Design review of the part built by this model. Coordinates are the model's own, in mm. A direction names the side the tool comes from. Give positions to 0.01 mm unless a question says otherwise; leave off trailing zeros. Write each loop counter-clockwise with the first axis right and the second up, starting at its lowest first coordinate (ties: lowest second). Pieces come first, ordered by that corner, then holes. Notation, with made-up numbers: (-8.5, 44) -> (47.5, 44) arc R15 cw to (47.5, 51) -> close; hole circle Ø5 at (59.5, -10.5). An arc over 180 degrees is marked (long way). Write each question's results on one line, items separated by ' | '. Start each with the question number.
(1) Take a section at B-B (y = -4.75). State the section outline as (x, z) points.
(2) Take a section at C-C (x = -2). State the section outline as (y, z) points, plus the area to 3 significant figures.
(3) Mouldability with a two-part tool opening along Y and no side actions: class faces 1 (the face through (-3.251, 5.455, 5.027)), 2 (the face through (-1.89, 10.15, 0)), 3 (the face through (11.81, 3.72, 5.01)) as released by +Y, released by -Y, zero draft, split by the parting line, or undercut.
(4) Clearance check with flat-ended pins moving along their axes: pin 1 (3 mm diameter, centred on x = 4, y = 4, fed in from +Z); pin 2 (4 mm diameter, centred on x = -5, z = 7, fed in from +Y); pin 3 (4 mm diameter, centred on x = -9, z = 4, fed in from -Y). State where each tip first meets the part, or that it passes through.
(5) Take a section at D-D (y = -9.25). State the section outline as (x, z) points.
(6) Take a section at A-A (z = 4.25). State the section outline as (x, y) points (1 decimal), plus the area to 3 significant figures.
(7) To check wall thickness, follow probe 1 along Y at (x, z) = (0, 0.9); probe 2 along X at (y, z) = (4.75, 8.5); probe 3 along Y at (x, z) = (4.25, 9.5). State the ranges of each line that lie inside material, in increasing order.
(8) For faces 4 (the face through (7, 0, 1.27)), 5 (the face through (-3.1, -5.54, 5.03)), 6 (the face through (-1.323, 10.074, 9.534)), list the 3-axis set-ups (+Z, -Z, +X, -X, +Y, -Y) from which the entire face can be reached by the end or side of a thin tool; tool diameter is ignored.
from build123d import *

# Parameters (mm, degrees)
SKETCH1_R               = 12.3825
BOSS_EXTRUDE1_DEPTH     = 10.16
ESQUISSE1_R             = 10.16
ENL_V_MAT_EXTRU_1_DEPTH = 1.27
ENL_V_START             = -1.27
ESQUISSE2_R             = 10.16
ENL_V_MAT_EXTRU_2_DEPTH = 1.27


with BuildPart() as part:
    # Sketch1 → Boss-Extrude1 (new body)
    with BuildSketch(Plane.XY):
        Circle(SKETCH1_R)
        Polygon((0.160352547, -7.330594819), (6.428657611, -3.52642803), (6.268305064, 3.804166789), (-0.160352547, 7.330594819), (-6.428657611, 3.52642803), (-6.268305064, -3.804166789), align=None, mode=Mode.SUBTRACT)
    extrude(amount=BOSS_EXTRUDE1_DEPTH)

    # Esquisse1 → Enlèv. mat.-Extru.1 (cut)
    with BuildSketch(Plane.XY.offset(10.16)):
        Circle(ESQUISSE1_R)
    extrude(amount=-ENL_V_MAT_EXTRU_1_DEPTH, mode=Mode.SUBTRACT)

    # Esquisse2 → Enlèv. mat.-Extru.2 (cut)
    with BuildSketch(Plane(origin=(0, 0, 0), x_dir=(-1, 0, 0), z_dir=(0, 0, -1)).offset(ENL_V_START)):
        with Locations(Location((0, 0, 0), (0, 0, 180))):
            Circle(ESQUISSE2_R)
    extrude(amount=ENL_V_MAT_EXTRU_2_DEPTH, mode=Mode.SUBTRACT)


solid = part.part
Report:
1) outline: (-11.44, 0) -> (-8.98, 0) -> (-8.98, 1.27) -> (-4.54, 1.27) -> (-4.54, 8.89) -> (-8.98, 8.89) -> (-8.98, 10.16) -> (-11.44, 10.16) -> close; (4.41, 1.27) -> (8.98, 1.27) -> (8.98, 0) -> (11.44, 0) -> (11.44, 10.16) -> (8.98, 10.16) -> (8.98, 8.89) -> (4.41, 8.89) -> close
2) outline: (-12.22, 0) -> (-9.96, 0) -> (-9.96, 1.27) -> (-6.15, 1.27) -> (-6.15, 8.89) -> (-9.96, 8.89) -> (-9.96, 10.16) -> (-12.22, 10.16) -> close; (6.21, 1.27) -> (9.96, 1.27) -> (9.96, 0) -> (12.22, 0) -> (12.22, 10.16) -> (9.96, 10.16) -> (9.96, 8.89) -> (6.21, 8.89) -> close | area: 104 mm2
3) face 1: undercut | face 2: zero draft | face 3: split by the parting line
4) pin 1: z = 8.89 | pin 2: y = 12.01 | pin 3: y = -10.21
5) outline: (-8.23, 0) -> (-4.2, 0) -> (-4.2, 1.27) -> (4.2, 1.27) -> (4.2, 0) -> (8.23, 0) -> (8.23, 10.16) -> (4.2, 10.16) -> (4.2, 8.89) -> (-4.2, 8.89) -> (-4.2, 10.16) -> (-8.23, 10.16) -> close
6) outline: circle Ø24.8 at (0, 0); hole (-6.4, 3.5) -> (-6.3, -3.8) -> (0.2, -7.3) -> (6.4, -3.5) -> (6.3, 3.8) -> (-0.2, 7.3) -> close | area: 342 mm2
7) probe 1: -12.38 to -10.16, 10.16 to 12.38 | probe 2: -11.44 to -4.41, 4.54 to 11.44 | probe 3: -11.63 to -9.23, 9.23 to 11.63
8) face 4: -Z | face 5: +Z, -Z | face 6: +Z
